Part model, mm, in its own coordinate system. Give positions to 0.01 mm unless a question says otherwise; leave off trailing zeros. Write each loop counter-clockwise with the first axis right and the second up, starting at its lowest first coordinate (ties: lowest second). Pieces come first, ordered by that corner, then holes. Notation, with made-up numbers: M 8.25,87 L 20.25,87 A13 ccw 20.25,93 Z; hole C -27,-27.5 d9. An arc over 180 degrees is marked long. Use a Markdown table: item, result. Add a question column.
from build123d import *

# Parameters (mm, degrees)
BOSS_EXTRUDE1_DEPTH      = 1
BOSS_EXTRUDE1_DEPTH_BACK = 1.3622
SKETCH15_R               = 1.6
CUT_EXTRUDE1_DEPTH       = 10


with BuildPart() as part:
    # Sketch1 → Boss-Extrude1 (new, two sides: drawn at the far end of the back side and taken through both)
    with BuildSketch(Plane(origin=(0, 0, 0), x_dir=(1, 0, 0), z_dir=(0, 1, 0)).offset(-BOSS_EXTRUDE1_DEPTH_BACK)):
        with BuildLine():
            Line((-8.087993737, -17.857854423), (20.396582526, -17.857854423))
            Line((20.396582526, -17.857854423), (20.396582526, -86.127406927))
            Line((20.396582526, -86.127406927), (-8.087993737, -86.127406927))
            add(Edge.make_bspline(
                [(-8.087993737, -17.857854423), (-19.823523703, -38.981015745), (-18.062835517, -64.98565312), (-8.087993737, -86.127406927)],
                knots=[0, 0, 0, 0, 1, 1, 1, 1], degree=3))
        make_face()
    extrude(amount=BOSS_EXTRUDE1_DEPTH + BOSS_EXTRUDE1_DEPTH_BACK)

    # Sketch15 → Cut-Extrude1 (cut)
    with BuildSketch(Plane(origin=(0, 1, 0), x_dir=(1, 0, 0), z_dir=(0, 1, 0))):
        with Locations(Location((-5.527632766, -22.423505535, 0), (0, 0, 270))):
            Circle(SKETCH15_R)
        with Locations(Location((16.472367234, -22.423505535, 0), (0, 0, 270))):
            Circle(SKETCH15_R)
        with Locations(Location((-5.527632766, -82.423505535, 0), (0, 0, 270))):
            Circle(SKETCH15_R)
        with Locations(Location((16.472367234, -82.423505535, 0), (0, 0, 270))):
            Circle(SKETCH15_R)
        with Locations(Location((-5.527632766, -74.423505535, 0), (0, 0, 270))):
            Circle(SKETCH15_R)
        with Locations(Location((16.472367234, -74.423505535, 0), (0, 0, 270))):
            Circle(SKETCH15_R)
        with Locations(Location((-5.527632766, -28.423505535, 0), (0, 0, 270))):
            Circle(SKETCH15_R)
    extrude(amount=-CUT_EXTRUDE1_DEPTH, mode=Mode.SUBTRACT)


solid = part.part
1. Cut at B-B (y = -0.4). Give the number of separate pieces and of enclosed holes in the cut face, then the cut area to 3 significant figures.
2. Mould opens along X. For faces 1 (the flat face through (5, 1, 52)), 2 (the cylindrical face through (-5.05, -0.16, 75.95)), 3 (the cylindrical face through (16.95, -0.16, 23.95)), 4 (the flat face through (20.397, 0, 52)) say: released by +X, released by -X, zero draft, split by the parting line, or undercut.
3. Drill centre lines: probe 1 along Z at (x, y) = (-5.5, 0.4); probe 2 along Z at (x, y) = (17, -1.05); probe 3 along Z at (x, y) = (16, 0.45). Where is each one in solid material? Low to high. Write a range as [from, to].
4. Cut at A-A (x = -6.5). Write the cut outline in (y, z), then the cut area to 3 significant figures.
A:
| question | item | result |
|---|---|---|
| 1 | separate pieces | 1 |
| 1 | enclosed holes | 7 |
| 1 | area | 2,260 mm² |
| 2 | face 1 | zero draft |
| 2 | face 2 | undercut |
| 2 | face 3 | undercut |
| 2 | face 4 | released by +X |
| 3 | probe 1 | z = [17.86, 20.82], [24.02, 26.82], [30.02, 72.82], [76.02, 80.82], [84.02, 86.13] |
| 3 | probe 2 | z = [17.86, 20.91], [23.93, 72.91], [75.93, 80.91], [83.93, 86.13] |
| 3 | probe 3 | z = [17.86, 20.89], [23.95, 72.89], [75.95, 80.89], [83.95, 86.13] |
| 4 | outline | M -1.36,17.86 L 1,17.86 L 1,21.15 L -1.36,21.15 Z; M -1.36,23.69 L 1,23.69 L 1,27.15 L -1.36,27.15 Z; M -1.36,29.69 L 1,29.69 L 1,73.15 L -1.36,73.15 Z; M -1.36,75.69 L 1,75.69 L 1,81.15 L -1.36,81.15 Z; M -1.36,83.69 L 1,83.69 L 1,86.13 L -1.36,86.13 Z |
| 4 | area | 137 mm² |
